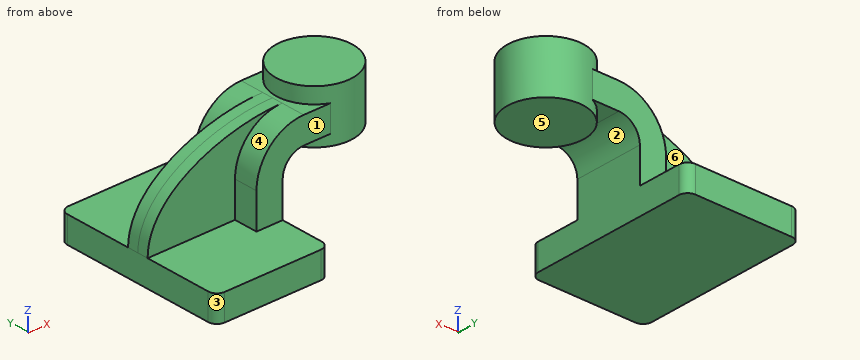
from build123d import *

# Parameters (mm, degrees)
F1_DEPTH = 63.5
F2_DEPTH = 25.4
F3_DEPTH = 7.9375
F5_R     = 6.35


with BuildPart() as f1:
    # F0 (on Front) → F1 (new body, symmetric)
    with BuildSketch(Plane.XZ):
        Polygon((41.275, -9.525), (41.275, 9.525), (22.225, 9.525), (-41.275, 9.525), (-41.275, -9.525), align=None)
    extrude(amount=F1_DEPTH, both=True)

    # F0 (on Front) → F2 (join, symmetric)
    with BuildSketch(Plane.XZ):
        with BuildLine():
            Line((22.225, 9.525), (41.275, 9.525))
            Line((41.275, 9.525), (41.275, 34.925))
            ThreePointArc((41.275, 34.925), (45.738693, 45.701307), (56.515, 50.165))
            Line((56.515, 50.165), (76.625528, 50.165))
            Line((76.625528, 50.165), (76.625528, 69.215))
            Line((76.625528, 69.215), (56.515, 69.215))
            ThreePointArc((56.515, 69.215), (32.268308, 59.171692), (22.225, 34.925))
            Line((22.225, 34.925), (22.225, 9.525))
        make_face()
    extrude(amount=F2_DEPTH, both=True)

    # F0 (on Front) → F3 (join, symmetric)
    with BuildSketch(Plane.XZ):
        with BuildLine():
            Line((-41.275, 9.525), (22.225, 9.525))
            Line((22.225, 9.525), (22.225, 34.925))
            ThreePointArc((22.225, 34.925), (32.268308, 59.171692), (56.515, 69.215))
            add(Edge.make_bspline(
                [(-41.275, 9.525), (-41.123904, 48.20979), (14.377582, 69.315985), (56.515, 69.215)],
                knots=[0, 0, 0, 0, 114.567797, 114.567797, 114.567797, 114.567797], degree=3))
        make_face()
    extrude(amount=F3_DEPTH, both=True)

    # F0 (on Front) → F4 (revolve)
    with BuildSketch(Plane.XZ):
        Polygon((86.995, 69.215), (86.995, 50.165), (86.995, 42.44888), (114.725528, 42.44888), (114.725528, 80.54888), (86.995, 80.54888), align=None)
    revolve(axis=Axis((86.995, 0, 61.49888), (0, 0, -1)))

    # F5
    f5_edges = [f1.edges().sort_by_distance(p)[0] for p in [
        (-41.275, 63.5, 0),
        (-41.275, -63.5, 0),
        (41.275, 63.5, 0),
        (41.275, -63.5, 0),
    ]]
    fillet(f5_edges, radius=F5_R)


solid = f1.part
Verification items for the finished model (mm, model axes). Face numbers are marked on the shaded views. A direction names the side the tool comes from. Round coordinates to 2 decimals unless told otherwise and drop trailing zeros. Loops run counter-clockwise (first coordinate to the right, second up) from the corner with the lowest first, then second, coordinate; pieces in that order, holes last. Notation, with made-up numbers: (56.25, 32) - (62.25, 32) arc R11 ccw to (62.25, 36) - close; hole circle Ø10 at (76.5, 11). An arc over 180 degrees is marked (long way). Use a Markdown table: item, result. Add a question column.
1. Section check C-C, the plane x = 101.5. Record the boundary of the cut face in (y, z), plus the area to 3 significant figures.
2. Section check B-B, the plane z = 75. Record the boundary of the cut face in (x, y) (3 decimals).
3. Gauge pin test, flat ends, axial feed: pin 1 (10 mm diameter, centred on x = 70, y = 8, fed in from -Z); pin 2 (4 mm diameter, centred on x = -14, z = 40, fed in from +Y); pin 3 (3 mm diameter, centred on x = 36, z = 14.5, fed in from +Y). Record the tip position at first contact, or that the pin passes through.
4. Section check D-D, the plane y = -54.5. Record the boundary of the cut face in (x, z) (3 decimals), plus the area to 3 significant figures.
5. Section check A-A, the plane y = -18. Record the boundary of the cut face in (x, z) (3 decimals), plus the area to 3 significant figures.
6. Thickness scan on probe 1 along X at (y, z) = (-12, 35.5); probe 2 along Y at (x, z) = (33.5, 33.5); probe 3 along Z at (x, y) = (61, -21) (3 decimals). Record the ranges inside material, lowest first. Write a range as [from, to].
7. Release check for a two-part mould opening along X. For the marked faces 1, 2 and 3 record: released by +X, released by -X, zero draft, split by the parting line, or undercut.
8. Access from +Z, -Z, +X, -X, +Y, -Y to the whole of each face (thin tool, end or side, straight path). Record for the marked faces 4, 5 and 6.
Checks:
| question | item | result |
|---|---|---|
| 1 | outline | (-23.63, 42.45) - (23.63, 42.45) - (23.63, 80.55) - (-23.63, 80.55) - close |
| 1 | area | 1,800 mm^2 |
| 2 | outline | circle Ø55.461 at (86.995, 0) |
| 3 | pin 1 | stops at z = 42.45 |
| 3 | pin 2 | stops at y = 7.94 |
| 3 | pin 3 | stops at y = 25.4 |
| 4 | outline | (-41.275, -9.525) - (41.275, -9.525) - (41.275, 9.525) - (-41.275, 9.525) - close |
| 4 | area | 1,570 mm^2 |
| 5 | outline | (-41.275, -9.525) - (41.275, -9.525) - (41.275, 34.925) arc R15.24 cw to (56.515, 50.165) - (65.9, 50.165) - (65.9, 42.449) - (108.09, 42.449) - (108.09, 80.549) - (65.9, 80.549) - (65.9, 69.215) - (56.515, 69.215) arc R34.29 ccw to (22.225, 34.925) - (22.225, 9.525) - (-41.275, 9.525) - close |
| 5 | area | 4,580 mm^2 |
| 6 | probe 1 | x = [22.23, 41.29] |
| 6 | probe 2 | y = [-25.4, 25.4] |
| 6 | probe 3 | z = [50.165, 69.215] |
| 7 | face 1 | zero draft |
| 7 | face 2 | undercut |
| 7 | face 3 | released by -X |
| 8 | face 4 | +Z, -X, -Y |
| 8 | face 5 | -Z, +X, +Y, -Y |
| 8 | face 6 | +Z, -X, +Y |
